The model under review builds one solid part; all positions refer to its coordinate system, in mm. Face numbers are marked on the shaded views. A direction names the side the tool comes from. Round coordinates to 2 decimals unless told otherwise and drop trailing zeros. Order: outer loops, then holes, each group sorted by start corner. A loop starts at its lowest first (then second) coordinate and runs counter-clockwise, first axis right, second up. Notation, with made-up numbers: M 45,71.5 L 103,71.5 A29 ccw 103,94.5 Z; hole C -4,19.25 d2. An arc over 180 degrees is marked long. Use a Markdown table: item, result. Add a question column.
1. For the marked faces 3 and 4, list the 3-axis set-ups (+Z, -Z, +X, -X, +Y, -Y) from which the entire face can be reached by the end or side of a thin tool; tool diameter is ignored.
2. Consider section B-B on y = -36.5. State the section outline as (x, z) points.
3. The part is to be moulded in two halves that separate along Z. For the marked faces 1 and 2, say which applies: +Z half, -Z half, draft (parallel to the pull), parting line (faces both ways), or undercut.
4. Consider section C-C on x = 55. State the section outline as (y, z) points.
5. Consider section A-A on z = 0. State the section outline as (x, y) points, then the cut area to 4 significant figures.
6. Insertion check: P1, Ø4, axis at x = 4, z = -17.5, coming from the +Y side; P2, Ø6, axis at x = 40.5, y = -4.5, coming from the -Z side; P3, Ø12, axis at x = 3, y = -10.5, coming from the +Z side. Each pin has a flat end and moves straight along its axis. Give the tip position at first contact, or say it passes through.
7. To check wall thickness, follow probe 1 along X at (y, z) = (-30, 0). State the ranges of the line that lie inside material, in increasing order.
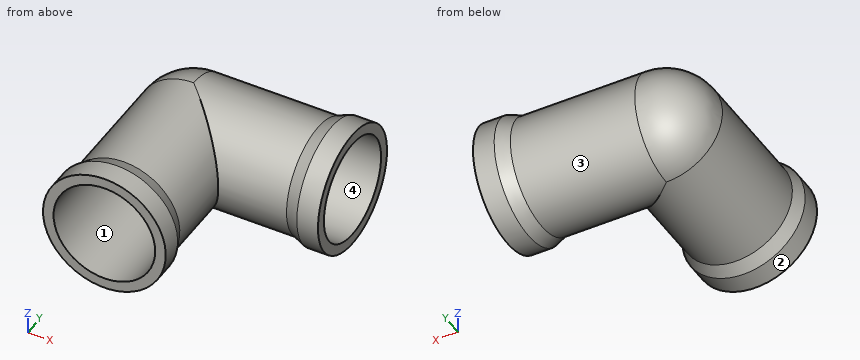
from build123d import *

# Parameters (mm, degrees)
SKETCH001_R          = 19.2
POCKET_DEPTH         = 60.001
POCKET001_DEPTH      = 23.201
POCKET001_DEPTH_BACK = -23.201
REVOLUTION001_ANGLE  = 90
SKETCH004_R          = 19.2
POCKET002_DEPTH      = 64


with BuildPart() as part:
    # Sketch → Revolution (revolve)
    with BuildSketch(Plane.XZ):
        Polygon((0, 0), (0, 21.2), (47, 21.2), (52, 23.2), (60, 23.2), (60, 0), align=None)
    revolve(axis=Axis((0, 0, 0), (1, 0, 0)))

    # Sketch001 (on Face5 of Revolution) → Pocket (cut, through all)
    with BuildSketch(Plane(origin=(60, 0, 0), x_dir=(0, 0, 1), z_dir=(1, 0, 0))):
        Circle(SKETCH001_R)
    extrude(amount=-POCKET_DEPTH, mode=Mode.SUBTRACT)

    # Sketch002 → Pocket001 (cut, two sides)
    with BuildSketch(Plane.XY) as pocket001_sk:
        Polygon((0, 0), (35.582964, -35.582964), (0, -35.582964), align=None)
    extrude(amount=-POCKET001_DEPTH, mode=Mode.SUBTRACT)
    extrude(pocket001_sk.sketch, amount=-POCKET001_DEPTH_BACK, mode=Mode.SUBTRACT)

    # Pocket001 Face1 → Revolution001 (revolve)
    with BuildSketch(Plane(origin=(0, 12.870225, 0), x_dir=(0, 1, 0), z_dir=(-1, 0, 0))):
        with BuildLine():
            Line((-12.870225, -19.2), (-12.870225, -21.2))
            ThreePointArc((-12.870225, -21.2), (8.329775, 0), (-12.870225, 21.2))
            Line((-12.870225, 21.2), (-12.870225, 19.2))
            ThreePointArc((-12.870225, 19.2), (6.329775, 0), (-12.870225, -19.2))
        make_face()
    revolve(axis=Axis((0, 0, 0), (0, 0, 1)), revolution_arc=REVOLUTION001_ANGLE)

    # Sketch003 → Revolution002 (revolve)
    with BuildSketch(Plane(origin=(0, 0, 0), x_dir=(0, -1, 0), z_dir=(-1, 0, 0))):
        Polygon((0, 0), (0, 21.2), (47, 21.2), (52, 23.2), (60, 23.2), (60, 0), align=None)
    revolve(axis=Axis((0, 0, 0), (0, -1, 0)))

    # Sketch004 (on Face9 of Revolution002) → Pocket002 (cut)
    with BuildSketch(Plane.XZ.offset(60)):
        Circle(SKETCH004_R)
    extrude(amount=-POCKET002_DEPTH, mode=Mode.SUBTRACT)


solid = part.part
Answer block:
| question | item | result |
|---|---|---|
| 1 | face 3 | none |
| 1 | face 4 | +X |
| 2 | outline | C 0,0 d42.4; hole C 0,0 d38.4 |
| 3 | face 1 | undercut |
| 3 | face 2 | parting line |
| 4 | outline | C 0,0 d46.4; hole C 0,0 d38.4 |
| 5 | outline | M -23.2,-60 L -19.2,-60 L -19.2,4 L -18.78,4 A19.2 cw 0,19.2 L 60,19.2 L 60,23.2 L 52,23.2 L 47,21.2 L 0,21.2 A21.2 ccw -21.2,0 L -21.2,-47 L -23.2,-52 Z; M 19.2,-60 L 23.2,-60 L 23.2,-52 L 21.2,-47 L 21.2,-21.2 L 47,-21.2 L 52,-23.2 L 60,-23.2 L 60,-19.2 L 21.2,-19.2 L 21.2,0 L 19.2,0 Z |
| 5 | area | 584.5 mm^2 |
| 6 | P1 | y = 14.46 |
| 6 | P2 | z = -21.15 |
| 6 | P3 | z = 21.2 |
| 7 | probe 1 | -21.2 to -19.2, 19.2 to 21.2 |
